The drawing under review shows one solid part. Ordinate dimensions are in mm from its lowest x, y, z. A direction names the side the tool comes from. Round coordinates to 2 decimals unless told otherwise and drop trailing zeros. Order: outer loops, then holes, each group sorted by start corner. A loop starts at its lowest first (then second) coordinate and runs counter-clockwise, first axis right, second up. Notation, with made-up numbers: (13.25, 26.5) -> (62.25, 26.5) arc R24 cw to (62.25, 56.5) -> close; hole circle Ø1 at (61, 82.25). An arc over 180 degrees is marked (long way). Put each result on its own line as item: value. Start each with the question number.
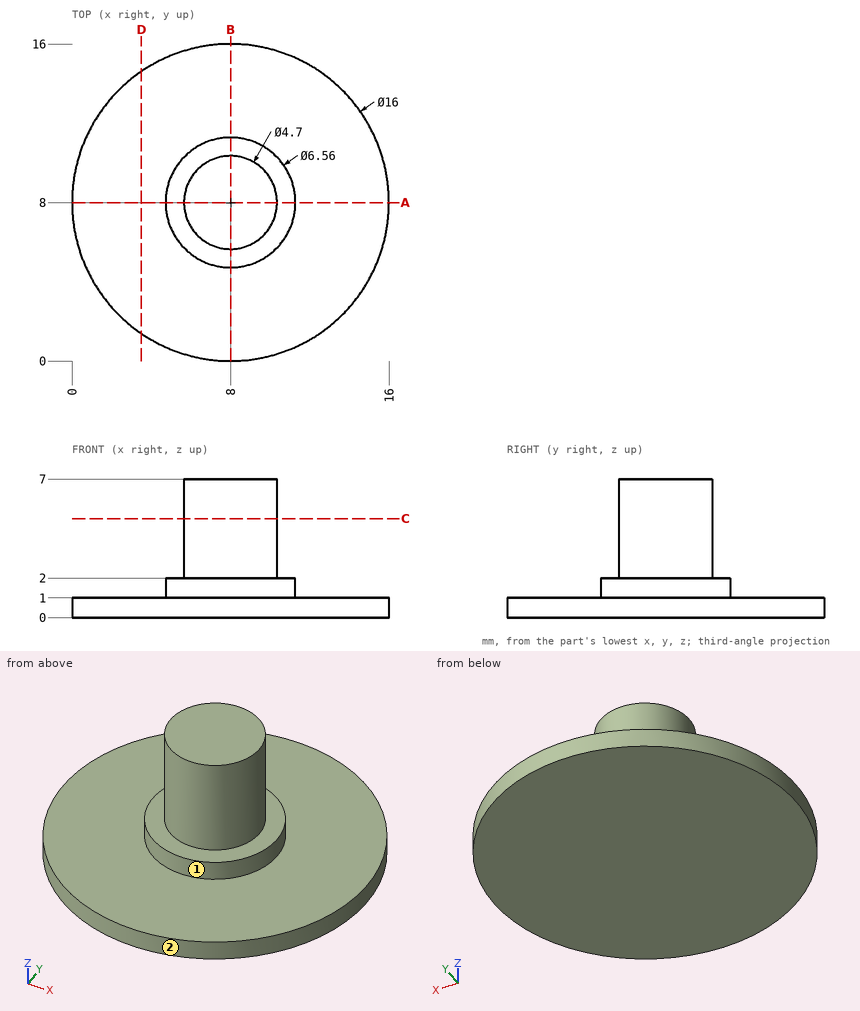
Item 1: Tool access review of the marked faces 1 and 2: name each direction out of +Z, -Z, +X, -X, +Y, -Y from which nothing blocks a thin tool from reaching the whole face with its end or side.
Item 2: For L1, parallel to Z at x = 9, y = 15; L2, parallel to X at y = 6.25, z = 2.75; L3, parallel to Y at x = 10.25, z = 0.75, list the stretches that pass through material, from the lowest coordinate up.
Item 3: Consider section C-C, the plane z = 5. Write out the cut boundary in (x, y).
Item 4: Insertion check: pin 1 Ø1.5 at (x, y) = (10.5, 4) entering from +Z; pin 2 Ø1.5 at (y, z) = (13.5, 1) entering from -X; pin 3 Ø3 at (x, z) = (7, 6) entering from -Y. Each pin has a flat end and moves straight along its axis. Give the tip position at first contact, or say it passes through.
Item 5: Consider section A-A, the plane y = 8. Write out the cut boundary in (x, z).
Item 6: Consider section D-D, the plane x = 3.5. Write out the cut boundary in (y, z) (1 decimal).
Evaluation:
1. face 1: +Z
1. face 2: +Z, -Z
2. L1: z = 0 to 1
2. L2: x = 6.43 to 9.57
2. L3: y = 0.32 to 15.68
3. outline: circle Ø4.7 at (8, 8)
4. pin 1: stops at z = 1
4. pin 2: stops at x = 1.56
4. pin 3: stops at y = 5.65
5. outline: (0, 0) -> (16, 0) -> (16, 1) -> (11.28, 1) -> (11.28, 2) -> (10.35, 2) -> (10.35, 7) -> (5.65, 7) -> (5.65, 2) -> (4.72, 2) -> (4.72, 1) -> (0, 1) -> close
6. outline: (1.4, 0) -> (14.6, 0) -> (14.6, 1) -> (1.4, 1) -> close
